Geometry: final body of the model. Coordinates: model frame, mm. A direction names the side the tool comes from. Coordinates: 2 decimals unless noted, no trailing zeros. Write each loop counter-clockwise with the first axis right and the second up, starting at its lowest first coordinate (ties: lowest second). Pieces come first, ordered by that corner, then holes.
from build123d import *

# Parameters (mm, degrees)
SKETCH_W     = 42.3
SKETCH_H     = 48.3
SKETCH_R     = 1.25
SKETCH_R_2   = 12
PAD_DEPTH    = 3
SKETCH001_W  = 42.3
SKETCH001_H  = 3
PAD001_DEPTH = 34
SKETCH002_R  = 1.5
POCKET_DEPTH = 48.301


with BuildPart() as part:
    # Sketch → Pad (new body)
    with BuildSketch(Plane.XY):
        with Locations((21.15, 24.15)):
            Rectangle(SKETCH_W, SKETCH_H)
        with Locations((5.65, 36.65)):
            Circle(SKETCH_R, mode=Mode.SUBTRACT)
        with Locations((36.65, 36.65)):
            Circle(SKETCH_R, mode=Mode.SUBTRACT)
        with Locations((5.65, 5.65)):
            Circle(SKETCH_R, mode=Mode.SUBTRACT)
        with Locations((36.65, 5.65)):
            Circle(SKETCH_R, mode=Mode.SUBTRACT)
        with Locations((21.15, 21.15)):
            Circle(SKETCH_R_2, mode=Mode.SUBTRACT)
    extrude(amount=PAD_DEPTH)

    # Sketch001 → Pad001 (new body)
    with BuildSketch(Plane(origin=(0, 0, 0), x_dir=(1, 0, 0), z_dir=(0, 0, -1))):
        with Locations((21.15, -46.8)):
            Rectangle(SKETCH001_W, SKETCH001_H)
    extrude(amount=PAD001_DEPTH)

    # Sketch002 → Pocket (cut, through all)
    with BuildSketch(Plane(origin=(0, 48.3, 0), x_dir=(-1, 0, 0), z_dir=(0, 1, 0))):
        with Locations((-30.2, -8)):
            Circle(SKETCH002_R)
        with Locations((-12.1, -8)):
            Circle(SKETCH002_R)
        with Locations((-30.2, -26)):
            Circle(SKETCH002_R)
        with Locations((-12.1, -26)):
            Circle(SKETCH002_R)
    extrude(amount=-POCKET_DEPTH, mode=Mode.SUBTRACT)


solid = part.part
Item 1: Section B-B, the plane y = 36.65. Output: boundary loops of the cut face in (x, z), plus the area to 3 significant figures.
Derived:
outline: (0, 0) - (4.4, 0) - (4.4, 3) - (0, 3) - close; (6.9, 0) - (35.4, 0) - (35.4, 3) - (6.9, 3) - close; (37.9, 0) - (42.3, 0) - (42.3, 3) - (37.9, 3) - close
area: 112 mm2
Item 2: Section D-D, the plane y = 21.15. Output: boundary loops of the cut face in (x, z).
Derived:
outline: (0, 0) - (9.15, 0) - (9.15, 3) - (0, 3) - close; (33.15, 0) - (42.3, 0) - (42.3, 3) - (33.15, 3) - close
Item 3: Pull-direction query (Z, two-part tool) for faces 1 (the cylindrical face through (13.21, 46.82, -24.99)), 2 (the flat face through (21, 35, 3)), 3 (the cylindrical face through (9.16, 21.68, 1.48)); classes: released by +Z, released by -Z, zero draft, split by the parting line, or undercut.
Derived:
face 1: undercut
face 2: released by +Z
face 3: zero draft
Item 4: Section C-C, the plane x = 21.5. Output: boundary loops of the cut face in (y, z).
Derived:
outline: (0, 0) - (9.16, 0) - (9.16, 3) - (0, 3) - close; (33.14, 0) - (45.3, 0) - (45.3, -34) - (48.3, -34) - (48.3, 3) - (33.14, 3) - close
Item 5: Section A-A, the plane z = -8. Output: boundary loops of the cut face in (x, y), plus the area to 3 significant figures.
Derived:
outline: (0, 45.3) - (10.6, 45.3) - (10.6, 48.3) - (0, 48.3) - close; (13.6, 45.3) - (28.7, 45.3) - (28.7, 48.3) - (13.6, 48.3) - close; (31.7, 45.3) - (42.3, 45.3) - (42.3, 48.3) - (31.7, 48.3) - close
area: 109 mm2
Item 6: Material intervals for probe 1 along Z at (x, y) = (12, 46); probe 2 along Y at (x, z) = (21, 1); probe 3 along X at (y, z) = (36, 1), sorted ascending.
Derived:
probe 1: z = -34 to -27.5, -24.5 to -9.5, -6.5 to 3
probe 2: y = 0 to 9.15, 33.15 to 48.3
probe 3: x = 0 to 4.58, 6.72 to 35.58, 37.72 to 42.3
Item 7: Pin query (flat end, axial travel): pin 1 (1.8 mm diameter, centred on x = 30.2, z = -8, fed in from +Y); pin 2 (10 mm diameter, centred on x = 8.5, y = 17.5, fed in from -Z); pin 3 (3 mm diameter, centred on x = 5.65, y = 36.65, fed in from +Z); pin 4 (4 mm diameter, centred on x = 12.1, z = -8, fed in from -Y). Return the tip coordinate at first contact, or that it passes through.
Derived:
pin 1: passes through
pin 2: stops at z = 0
pin 3: stops at z = 3
pin 4: stops at y = 45.3
Item 8: Set-up query: faces 4 (the flat face through (21, 48.3, -15)), 5 (the flat face through (21, 45.3, -17)). Return all of +Z, -Z, +X, -X, +Y, -Y with unobstructed straight access to the full face (end or side cutting, diameter ignored); none if empty.
Derived:
face 4: +Z, -Z, +X, -X, +Y
face 5: -Z, +X, -X, -Y
